Geometry check sheet. Reference: the model listing, model coordinates, mm. Face numbers are marked on the shaded views. A direction names the side the tool comes from. Round coordinates to 2 decimals unless told otherwise and drop trailing zeros. Order: outer loops, then holes, each group sorted by start corner. A loop starts at its lowest first (then second) coordinate and runs counter-clockwise, first axis right, second up. Notation, with made-up numbers: M 88.25,28.25 L 128.25,28.25 A18 ccw 128.25,62.25 Z; hole C -29,58 d10. An arc over 180 degrees is marked long. Answer as a JSON object with one key per item and string values. Group by question number.
```python
from build123d import *

# Parameters (mm, degrees)
SKETCH1_W           = 55
SKETCH1_H           = 75
BOSS_EXTRUDE1_DEPTH = 30
SKETCH2_R           = 21.25
CUT_EXTRUDE1_DEPTH  = 30
SKETCH3_W           = 41
SKETCH3_H           = 16
CUT_EXTRUDE2_DEPTH  = 60
SKETCH4_W           = 16
SKETCH4_H           = 61
CUT_EXTRUDE3_DEPTH  = 60
SKETCH5_R           = 2.125
CUT_EXTRUDE4_DEPTH  = 10


with BuildPart() as part:
    # Sketch1 → Boss-Extrude1 (new body)
    with BuildSketch(Plane.XY):
        with Locations((0, 10)):
            Rectangle(SKETCH1_W, SKETCH1_H)
    extrude(amount=BOSS_EXTRUDE1_DEPTH)

    # Sketch2 → Cut-Extrude1 (cut)
    with BuildSketch(Plane.XY.offset(30)):
        Circle(SKETCH2_R)
    extrude(amount=-CUT_EXTRUDE1_DEPTH, mode=Mode.SUBTRACT)

    # Sketch3 → Cut-Extrude2 (cut)
    with BuildSketch(Plane(origin=(0, 47.5, 0), x_dir=(1, 0, 0), z_dir=(0, 1, 0))):
        with Locations((0, -15)):
            Rectangle(SKETCH3_W, SKETCH3_H)
    extrude(amount=-CUT_EXTRUDE2_DEPTH, mode=Mode.SUBTRACT)

    # Sketch4 → Cut-Extrude3 (cut)
    with BuildSketch(Plane(origin=(27.5, 0, 0), x_dir=(0, 0, -1), z_dir=(1, 0, 0))):
        with Locations((-15, 10)):
            Rectangle(SKETCH4_W, SKETCH4_H)
    extrude(amount=-CUT_EXTRUDE3_DEPTH, mode=Mode.SUBTRACT)

    # Sketch5 → Cut-Extrude4 (cut)
    with BuildSketch(Plane(origin=(0, 47.5, 0), x_dir=(1, 0, 0), z_dir=(0, 1, 0))):
        with Locations(Location((-24, -14, 0), (0, 0, 270))):
            Circle(SKETCH5_R)
        with Locations(Location((24, -14, 0), (0, 0, 270))):
            Circle(SKETCH5_R)
    extrude(amount=-CUT_EXTRUDE4_DEPTH, mode=Mode.SUBTRACT)


solid = part.part
```
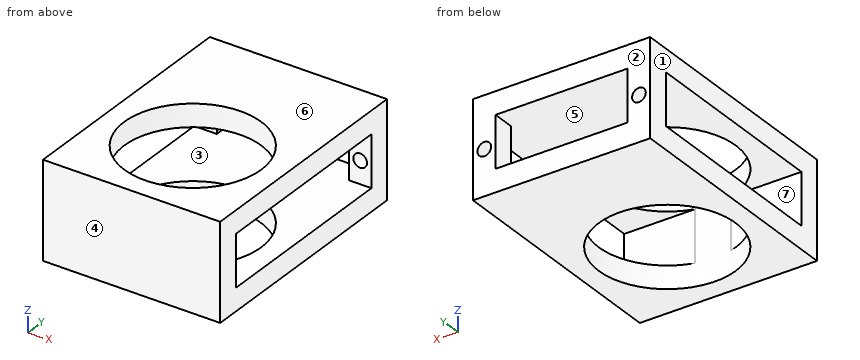
1) Go/stop test with a flat-tipped pin: P1, Ø1.5, axis at x = 19, z = 14, coming from the +Y side. Record where the tip stops, or that it passes through.
2) Sectioned sample at D-D (z = 26.5). Record the boundary of the cut face in (x, y), then the cut area to 3 significant figures.
3) Sectioned sample at C-C (x = 0). Record the boundary of the cut face in (y, z), then the cut area to 3 significant figures.
4) Release check for a two-part mould opening along Y. For the marked faces 1, 2, 3 and 4 record: +Y half, -Y half, draft (parallel to the pull), parting line (faces both ways), or undercut.
5) Sectioned sample at B-B (y = 33). Record the boundary of the cut face in (x, z).
6) Thickness scan on line 1 along X through (y, z) = (43.5, 14) (3 decimals); line 2 along Z through (x, y) = (19, -20); line 3 along X through (y, z) = (43, 21). Record the ranges inside material, lowest first. Write a range as [from, to].
7) Sectioned sample at A-A (z = 17). Record the boundary of the cut face in (x, y), then the cut area to 3 significant figures.
8) Set-up check for the marked faces 5, 6 and 7: record each of +Z, -Z, +X, -X, +Y, -Y from which the full face is reachable in a straight line by a thin tool's end or side.
Final values:
{
 "1": {"P1": "stops at y = -20.5"},
 "2": {"outline": "M -27.5,-27.5 L 27.5,-27.5 L 27.5,47.5 L -27.5,47.5 Z; hole C 0,0 d42.5", "area": "2,710 mm^2"},
 "3": {"outline": "M -27.5,0 L -21.25,0 L -21.25,30 L -27.5,30 Z; M 21.25,0 L 47.5,0 L 47.5,7 L 21.25,7 Z; M 21.25,23 L 47.5,23 L 47.5,30 L 21.25,30 Z", "area": "555 mm^2"},
 "4": {"face 1": "draft", "face 2": "+Y half", "face 3": "undercut", "face 4": "-Y half"},
 "5": {"outline": "M -27.5,0 L 27.5,0 L 27.5,7 L -27.5,7 Z; M -27.5,23 L 27.5,23 L 27.5,30 L -27.5,30 Z"},
 "6": {"line 1": "x = [-27.5, -26.125], [-21.875, -20.5], [20.5, 21.875], [26.125, 27.5]", "line 2": "z = [0, 7], [23, 30]", "line 3": "x = [-27.5, -20.5], [20.5, 27.5]"},
 "7": {"outline": "M -27.5,-27.5 L 27.5,-27.5 L 27.5,-20.5 L 5.6,-20.5 A21.25 cw -5.6,-20.5 L -27.5,-20.5 Z; M -27.5,40.5 L -20.5,40.5 L -20.5,47.5 L -27.5,47.5 Z; M 20.5,40.5 L 27.5,40.5 L 27.5,47.5 L 20.5,47.5 Z", "area": "477 mm^2"},
 "8": {"face 5": "none", "face 6": "+Z, +X, -X, +Y, -Y", "face 7": "+X, -X"}
}
